The model under review builds one solid part; all positions refer to its coordinate system, in mm. A direction names the side the tool comes from. Round coordinates to 2 decimals unless told otherwise and drop trailing zeros. Order: outer loops, then holes, each group sorted by start corner. A loop starts at its lowest first (then second) coordinate and runs counter-clockwise, first axis right, second up.
from build123d import *

# Parameters (mm, degrees)
F3_DEPTH = 20
F4_R     = 4.99999
F6_DEPTH = 2.6
F7_D     = 3.6
F7_DEPTH = 10
F7_TIP   = 1.0815491142
F8_R     = 34


# Not quite as in the source:
# - a fillet or chamfer is up to 0.001 mm smaller than in the source, because OpenCascade refuses the exact size


with BuildPart() as f3:
    # F2 (on Top) → F3 (new body)
    with BuildSketch(Plane.XY):
        Polygon((0, 5), (0, 0), (20, 0), (20, -22), (0, -22), (0, -27), (30, -27), (30, 0), (80, 0), (80, 15), (75, 15), (75, 5), align=None)
    extrude(amount=F3_DEPTH)

    # F4 (radius 5 in the source; OpenCascade refuses exactly that, so slightly less here)
    f4_edges = [f3.edges().sort_by_distance(p)[0] for p in [
        (30, -27, 10),
        (80, 0, 10),
        (80, 15, 10),
        (0, 5, 10),
        (0, -27, 10),
    ]]
    fillet(f4_edges, radius=F4_R)

    # F5 (on face) → F6 (cut)
    with BuildSketch(Plane(origin=(0, -22, 0), x_dir=(-1, 0, 0), z_dir=(0, 1, 0))):
        Polygon((-7.25, 8.4122867597), (-7.25, 11.5877132403), (-10, 13.1754264805), (-12.75, 11.5877132403), (-12.75, 8.4122867597), (-10, 6.8245735195), align=None)
    extrude(amount=-F6_DEPTH, mode=Mode.SUBTRACT)

    # F7 (one way)
    with BuildSketch(Plane(origin=(0, -22, 0), x_dir=(-1, 0, 0), z_dir=(0, 1, 0))):
        with Locations((-10, 10)):
            Circle(F7_D / 2)
    extrude(amount=-F7_DEPTH, mode=Mode.SUBTRACT)
    with Locations(Plane(origin=(0, -22, 0), x_dir=(-1, 0, 0), z_dir=(0, 1, 0))):
        with Locations((-10, 10)):
            with Locations((0, 0, -(F7_DEPTH + F7_TIP / 2))):  # 118° drill point
                Cone(0, F7_D / 2, F7_TIP, mode=Mode.SUBTRACT)

    # F8
    f8_edges = [f3.edges().sort_by_distance(p)[0] for p in [
        (30, 0, 10),
    ]]
    fillet(f8_edges, radius=F8_R)


solid = f3.part
(1) To check wall thickness, follow L1, parallel to Z at x = 10, y = -26; L2, parallel to X at y = 8.5, z = 12.5; L3, parallel to Y at x = 63, z = 14.5. State the ranges of each line that lie inside material, in increasing order.
(2) The part is to be moulded in two halves that separate along Z. For faces 5 (the flat face through (34, -6, 0)), 6 (the flat face through (7.25, -23, 10)), 7 (the flat face through (68, 0, 10)), say which applies: pulls with the +Z half, pulls with the -Z half, needs draft (parallel to the pull), parting line crosses it, or undercut.
(3) We need section B-B (y = 8). Give the boundary of the cut face in (x, z).
(4) We need section A-A (x = 18.5). Give the boundary of the cut face in (y, z), and give its area (3 significant figures).
(5) We need section C-C (x = 29). Give the boundary of the cut face in (y, z).
(6) Clearance check with flat-ended pins moving along their axes: P1, Ø4.5, axis at x = 10, z = 10, coming from the -Y side; P2, Ø6, axis at x = 9, z = 10.5, coming from the +Y side; P3, Ø3, axis at y = 11, z = 11.5, coming from the -X side; P4, Ø6, axis at y = -14.5, z = 18, coming from the -X side. State where each tip first meets the part, or that it passes through.
(7) Tool access review of faces 1 (the flat face through (40, 5, 10)), 2 (the flat face through (20, -11, 10)), 3 (the flat face through (11.394, -23.282, 7.63)), 4 (the cylindrical face through (10.39, -25.783, 8.243)): name each direction out of +Z, -Z, +X, -X, +Y, -Y from which nothing blocks a thin tool from reaching the whole face with its end or side.
Verdict:
1. L1: z = 0 to 8.2, 11.8 to 20
1. L2: x = 75 to 80
1. L3: y = 0 to 5
2. face 5: pulls with the -Z half
2. face 6: undercut
2. face 7: needs draft
3. outline: (75, 0) - (80, 0) - (80, 20) - (75, 20) - close
4. outline: (-27, 0) - (-22, 0) - (-22, 20) - (-27, 20) - close; (0, 0) - (5, 0) - (5, 20) - (0, 20) - close
4. area: 200 mm2
5. outline: (-25, 0) - (5, 0) - (5, 20) - (-25, 20) - close
6. P1: stops at y = -27
6. P2: stops at y = 5
6. P3: stops at x = 75
6. P4: stops at x = 20
7. face 1: +Z, -Z, -X, +Y
7. face 2: +Z, -Z, -X
7. face 3: none
7. face 4: -Y
